Geometry: final body of the model. Coordinates: model frame, mm. A direction names the side the tool comes from. Coordinates: 2 decimals unless noted, no trailing zeros. Loops run counter-clockwise (first coordinate to the right, second up) from the corner with the lowest first, then second, coordinate; pieces in that order, holes last. Notation, with made-up numbers: (70, -40) - (103, -40) arc R9 cw to (103, -31) - close; hole circle Ø11 at (60.25, 54). An arc over 180 degrees is marked (long way). Answer in a Markdown table with one row per item.
Autodesk Inventor part; units mm, degrees
ref_plane "YZ Plane" through (0, 0, 0) normal (1, 0, 0) x (0, 1, 0)
ref_plane "XZ Plane" through (0, 0, 0) normal (0, 1, 0) x (-1, 0, 0)
ref_plane "XY Plane" through (0, 0, 0) normal (0, 0, 1) x (1, 0, 0)
sketch "スケッチ1" plane through (0, 0, 0) normal (0, 1, 0) x (-1, 0, 0)
  line L0 (24, 0) -> (0, 0)
  line L1 (0, 0) -> (0, -26)
  line L2 (0, -26) -> (24, -26)
  line L3 (24, -26) -> (24, 0)
  circle A0 centre (24, -13) radius 13 construction
  circle A1 centre (24, -13) radius 12.5
  circle A2 centre (24, -13) radius 16
  point P0 (24, -25.5)
  point P1 (24, -0.5)
  point P2 (14.6726, 0)
  point P3 (14.6726, -26)
  dimension "d0" = 26
  dimension "d1" = 24
  dimension "d2" = 25
  dimension "d3" = 32
extrude "押し出し1" add sketch "スケッチ1" along normal blind 4 contours L3 A1 L2 A2 L0 | A2 L2 L1 L0 picked at (14.0879, -23.9339)
extrude "押し出し2" cut sketch "スケッチ1" along normal blind 2.2 contours L3 A1 L2 A2 L0 picked at (14.0879, -23.9339)
fillet "フィレット1" radius 1 4 edges at (-24, 3.1, -0.5) (-24, 3.1, 0) (-24, 3.1, -26) (-24, 3.1, -25.5)
sketch "スケッチ2" plane through (0, 4, 0) normal (0, 1, 0) x (1, 0, 0)
  circle A0 centre (-3, 2.5) radius 0.85 construction
  circle A1 centre (-3, 23.5) radius 0.85 construction
  circle A2 centre (-3, 2.5) radius 0.8
  circle A3 centre (-3, 23.5) radius 0.8
  point P0 (0, 0)
  dimension "d9" = 1.6
  dimension "d10" = 1.6
extrude "押し出し3" cut sketch "スケッチ2" against normal through all
sketch "スケッチ3" plane through (0, 4, 0) normal (0, 1, 0) x (1, 0, 0)
  circle A0 centre (-3, 2.5) radius 0.8
  circle A1 centre (-3, 23.5) radius 0.8
  circle A2 centre (-3, 2.5) radius 2
  circle A3 centre (-3, 23.5) radius 2
  point P0 (0, 0)
  dimension "d13" = 4
  dimension "d14" = 4
extrude "押し出し4" cut sketch "スケッチ3" against normal blind 2.5 contours A0 | A1 | A2 | A3
fillet "フィレット2" radius 2 2 edges at (0, 2, 0) (0, 2, -26)
properties part number "sholder_joint_cover"
(1) Cut plane D-D on z = -2.5. Output: boundary loops of the cut face in (x, y).
Verdict:
| item | result |
|---|---|
| outline | (-17.22, 2.2) - (-11.93, 2.2) - (-11.93, 0) - (-3.8, 0) - (-3.8, 1.5) - (-5, 1.5) - (-5, 4) - (-17.22, 4) - close; (-2.2, 0) - (0, 0) - (0, 4) - (-1, 4) - (-1, 1.5) - (-2.2, 1.5) - close |
(2) Access query for faces 1 (the face through (-3.434, 2.768, -0.548)), 2 (the face through (-6, 0, -13)), 3 (the face through (-11, 2.2, -13)). Directions: +Z, -Z, +X, -X, +Y, -Y. A direction counts if a zero-diameter tool reaches every point of the face in a straight line with its end or side. Return the directions, or none.
Verdict:
| item | result |
|---|---|
| face 1 | +Y |
| face 2 | +Z, -Z, +X, -X, -Y |
| face 3 | -X, -Y |
(3) First-contact query: pin 1 Ø5 at (x, z) = (-15, -17.5) entering from -Y. Flat tip, straight axial feed; report the tip coordinate or a pass-through.
Verdict:
| item | result |
|---|---|
| pin 1 | stops at y = 2.2 |
(4) Ray query, probe 1 along Z at (x, y) = (-3, 3.2); probe 2 along Z at (x, y) = (-3, 0.7); probe 3 along X at (y, z) = (2.5, -13). Return the intervals inside material, ascending.
Verdict:
| item | result |
|---|---|
| probe 1 | z = -26 to -25.5, -21.5 to -4.5, -0.5 to 0 |
| probe 2 | z = -26 to -24.3, -22.7 to -3.3, -1.7 to 0 |
| probe 3 | x = -11.5 to 0 |
(5) Cut plane A-A on y = 2.85. Output: boundary loops of the cut face in (x, z), then the cut area to 3 significant figures.
Verdict:
| item | result |
|---|---|
| outline | (-18.27, -24.11) arc R1 ccw to (-17.82, -26) - (-2, -26) arc R2 ccw to (0, -24) - (0, -2) arc R2 ccw to (-2, 0) - (-17.82, 0) arc R1 ccw to (-18.27, -1.89) arc R12.5 cw to start; hole circle Ø4 at (-3, -23.5); hole circle Ø4 at (-3, -2.5) |
| area | 342 mm² |
(6) Cut plane B-B on x = -3. Output: boundary loops of the cut face in (y, z), then the cut area to 3 significant figures.
Verdict:
| item | result |
|---|---|
| outline | (0, -26) - (4, -26) - (4, -25.5) - (1.5, -25.5) - (1.5, -24.3) - (0, -24.3) - close; (0, -22.7) - (1.5, -22.7) - (1.5, -21.5) - (4, -21.5) - (4, -4.5) - (1.5, -4.5) - (1.5, -3.3) - (0, -3.3) - close; (0, -1.7) - (1.5, -1.7) - (1.5, -0.5) - (4, -0.5) - (4, 0) - (0, 0) - close |
| area | 79.2 mm² |
(7) Pull-direction query (X, two-part tool) for faces 4 (the face through (-18.79, 3.09, -25.22)), 5 (the face through (-10, 2, -26)), 6 (the face through (-2, 1.5, -3)), 7 (the face through (0, 2, -13)); classes: pulls with the +X half, pulls with the -X half, needs draft (parallel to the pull), parting line crosses it, or undercut.
Verdict:
| item | result |
|---|---|
| face 4 | pulls with the -X half |
| face 5 | needs draft |
| face 6 | undercut |
| face 7 | pulls with the +X half |
(8) Cut plane C-C on x = -16.25. Output: boundary loops of the cut face in (y, z).
Verdict:
| item | result |
|---|---|
| outline | (2.2, -26) - (4, -26) - (4, -22.81) - (2.2, -22.81) - close; (2.2, -3.19) - (4, -3.19) - (4, 0) - (2.2, 0) - close |
